The model under review builds one solid part; all positions refer to its coordinate system, in mm. Face numbers are marked on the shaded views. A direction names the side the tool comes from. Give positions to 0.01 mm unless a question says otherwise; leave off trailing zeros. Order: outer loops, then holes, each group sorted by start corner. A loop starts at its lowest first (then second) coordinate and runs counter-clockwise, first axis right, second up.
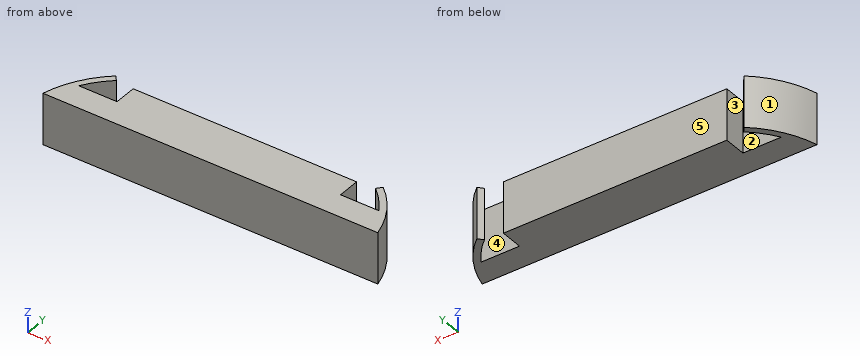
```python
from build123d import *

# Parameters (mm, degrees)
F1_DEPTH = 5.08


with BuildPart() as f1:
    # F0 (on Top) → F1 (new body)
    with BuildSketch(Plane.XY):
        with BuildLine():
            Line((0, 4.7625), (0, 0))
            Line((0, 0), (16.647249, 0))
            ThreePointArc((16.647249, 0), (15.405472, 2.967188), (13.298387, 5.3975))
            Line((13.298387, 5.3975), (12.8905, 4.910825))
            ThreePointArc((12.8905, 4.910825), (14.004311, 3.809245), (14.9225, 2.54))
            Line((14.9225, 2.54), (11.1125, 2.54))
            Line((11.1125, 2.54), (11.1125, 4.7625))
            Line((11.1125, 4.7625), (0, 4.7625))
        make_face()
    extrude(amount=F1_DEPTH)

    # F2: F1 across face


with BuildPart() as f1_1:
    add(f1.part)
    add(f1.part.mirror(Plane(origin=(0, 2.38125, 2.54), x_dir=(0, -1, 0), z_dir=(-1, 0, 0))))


solid = f1_1.part
```
Item 1: For the marked faces 1 and 2, list the 3-axis set-ups (+Z, -Z, +X, -X, +Y, -Y) from which the entire face can be reached by the end or side of a thin tool; tool diameter is ignored.
Values found:
face 1: +Z, -Z, -X, +Y
face 2: +Z, -Z
Item 2: Take a section at C-C (x = 5.5). Give the boundary of the cut face in (y, z).
Values found:
outline: (0, 0) - (4.76, 0) - (4.76, 5.08) - (0, 5.08) - close
Item 3: Take a section at B-B (z = 3.15). Give the boundary of the cut face in (x, y).
Values found:
outline: (-16.65, 0) - (16.65, 0) arc R10.16 ccw to (13.3, 5.4) - (12.89, 4.91) arc R9.53 cw to (14.92, 2.54) - (11.11, 2.54) - (11.11, 4.76) - (-11.11, 4.76) - (-11.11, 2.54) - (-14.92, 2.54) arc R9.53 cw to (-12.89, 4.91) - (-13.3, 5.4) arc R10.16 ccw to start
Item 4: Draft analysis for pull direction Y (two halves, no side actions). For the marked faces 3, 4 and 5, state which applies: released by +Y, released by -Y, zero draft, split by the parting line, or undercut.
Values found:
face 3: zero draft
face 4: undercut
face 5: released by +Y
Item 5: Clearance check with flat-ended pins moving along their axes: pin 1 Ø1.1 at (y, z) = (3.5, 3) entering from +X; pin 2 Ø3 at (y, z) = (2, 2.5) entering from +X; pin 3 Ø1.5 at (x, z) = (2.5, 2) entering from +Y. State where each tip first meets the part, or that it passes through.
Values found:
pin 1: stops at x = 15.42
pin 2: stops at x = 16.51
pin 3: stops at y = 4.76
Item 6: Take a section at D-D (y = 1.6). Give the boundary of the cut face in (x, z), and give its area (3 significant figures).
Values found:
outline: (-16.12, 0) - (16.12, 0) - (16.12, 5.08) - (-16.12, 5.08) - close
area: 164 mm2
Item 7: For line 1 (X direction, y = 2.95, z = 0.5); line 2 (X direction, y = 4.3, z = 4.55); line 3 (Y direction, x = 6, z = 4.5), list the stretches that pass through material, from the lowest coordinate up.
Values found:
line 1: x = -15.42 to -14.66, -11.11 to 11.11, 14.66 to 15.42
line 2: x = -14.42 to -13.55, -11.11 to 11.11, 13.55 to 14.42
line 3: y = 0 to 4.76
Item 8: Take a section at A-A (y = 3.95). Give the boundary of the cut face in (x, z), and give its area (3 significant figures).
Values found:
outline: (-14.71, 0) - (-13.88, 0) - (-13.88, 5.08) - (-14.71, 5.08) - close; (-11.11, 0) - (11.11, 0) - (11.11, 5.08) - (-11.11, 5.08) - close; (13.88, 0) - (14.71, 0) - (14.71, 5.08) - (13.88, 5.08) - close
area: 121 mm2
